For this review, use the dimensioned drawing (mm, ordinates from the lowest corner) and the shaded views. Give positions to 0.01 mm unless a question says otherwise; leave off trailing zeros. Order: outer loops, then holes, each group sorted by start corner. A loop starts at its lowest first (then second) coordinate and runs counter-clockwise, first axis right, second up.
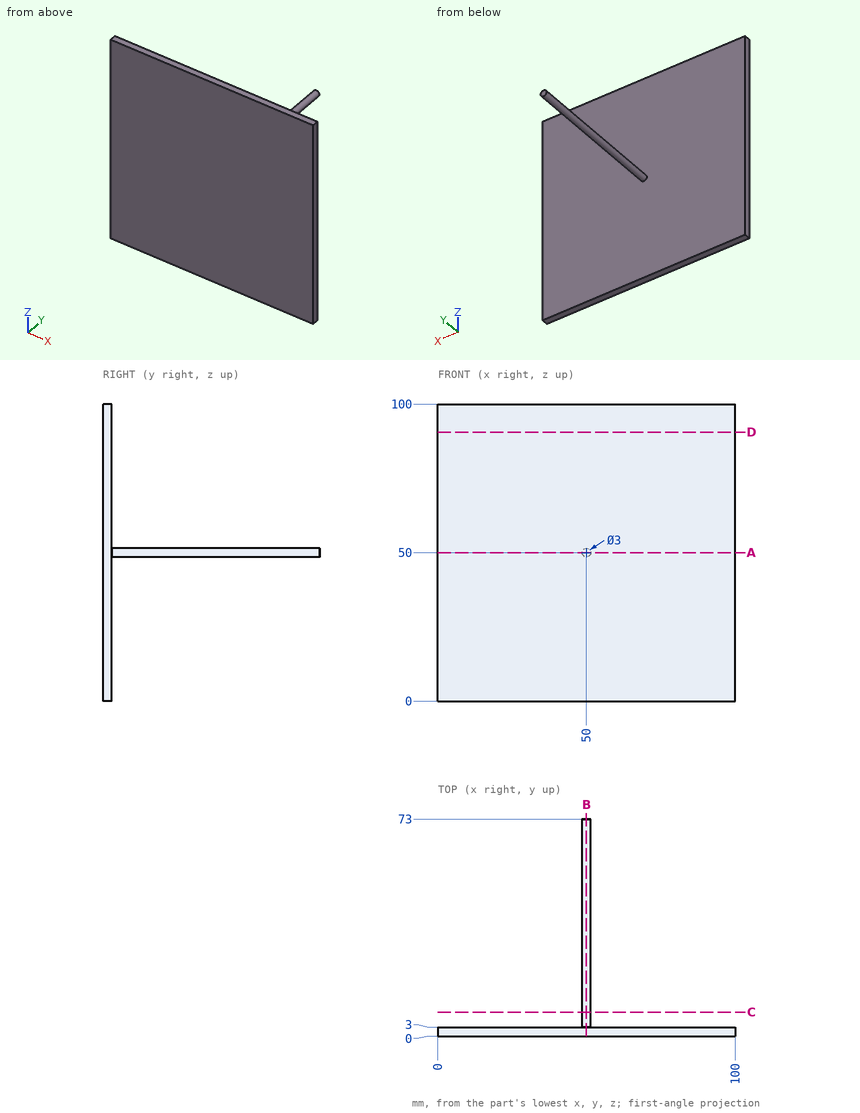
1. For line 1 along Y through (x, z) = (25.5, 29); line 2 along X through (y, z) = (22.5, 49.5), list the stretches that pass through material, from the lowest coordinate up.
Recorded:
line 1: y = 0 to 3
line 2: x = 48.59 to 51.41
2. Take a section at D-D (z = 90.5). State the section outline as (x, y) points.
Recorded:
outline: (0, 0) - (100, 0) - (100, 3) - (0, 3) - close
3. Take a section at A-A (z = 50). State the section outline as (x, y) points, then the cut area to 3 significant figures.
Recorded:
outline: (0, 0) - (100, 0) - (100, 3) - (51.5, 3) - (51.5, 73) - (48.5, 73) - (48.5, 3) - (0, 3) - close
area: 510 mm2
4. Take a section at C-C (y = 8). State the section outline as (x, z) points, then the cut area to 3 significant figures.
Recorded:
outline: circle Ø3 at (50, 50)
area: 7.07 mm2
5. Take a section at B-B (x = 50). State the section outline as (y, z) points.
Recorded:
outline: (0, 0) - (3, 0) - (3, 48.5) - (73, 48.5) - (73, 51.5) - (3, 51.5) - (3, 100) - (0, 100) - close
